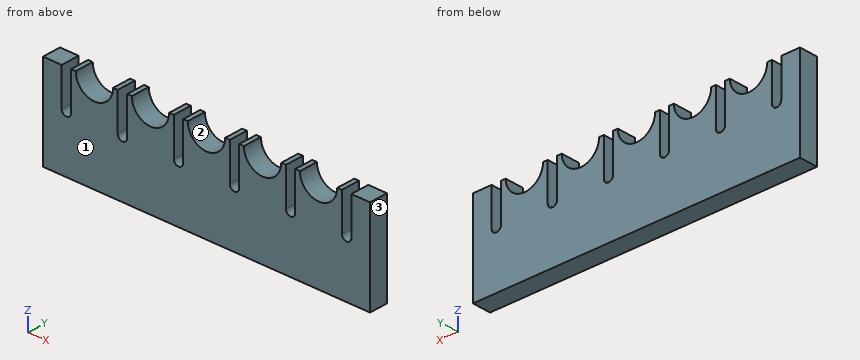
from build123d import *

# Parameters (mm, degrees)
BOSS_EXTRUDE1_DEPTH = 10


with BuildPart() as part:
    # Sketch2 → Boss-Extrude1 (new body)
    with BuildSketch(Plane(origin=(0, 0, 0), x_dir=(1, 0, 0), z_dir=(0, 1, 0))):
        with BuildLine():
            Line((-77.5, -25), (-77.5, -5))
            ThreePointArc((-77.5, -5), (-75, -2.5), (-72.5, -5))
            Line((-72.5, -5), (-72.5, -25))
            Line((-72.5, -25), (-70, -25))
            ThreePointArc((-70, -25), (-60, -15), (-50, -25))
            Line((-50, -25), (-47.5, -25))
            Line((-47.5, -25), (-47.5, -5))
            ThreePointArc((-47.5, -5), (-45, -2.5), (-42.5, -5))
            Line((-42.5, -5), (-42.5, -25))
            Line((-42.5, -25), (-40, -25))
            ThreePointArc((-40, -25), (-30, -15), (-20, -25))
            Line((-20, -25), (-17.5, -25))
            Line((-17.5, -25), (-17.5, -5))
            ThreePointArc((-17.5, -5), (-15, -2.5), (-12.5, -5))
            Line((-12.5, -5), (-12.5, -25))
            Line((-12.5, -25), (-10, -25))
            ThreePointArc((-10, -25), (0, -15), (10, -25))
            Line((10, -25), (12.5, -25))
            Line((12.5, -25), (12.5, -5))
            ThreePointArc((12.5, -5), (15, -2.5), (17.5, -5))
            Line((17.5, -5), (17.5, -25))
            Line((17.5, -25), (20, -25))
            ThreePointArc((20, -25), (30, -15), (40, -25))
            Line((40, -25), (42.5, -25))
            Line((42.5, -25), (42.5, -5))
            ThreePointArc((42.5, -5), (45, -2.5), (47.5, -5))
            Line((47.5, -5), (47.5, -25))
            Line((47.5, -25), (50, -25))
            ThreePointArc((50, -25), (60, -15), (70, -25))
            Line((70, -25), (72.5, -25))
            Line((72.5, -25), (72.5, -5))
            ThreePointArc((72.5, -5), (75, -2.5), (77.5, -5))
            Line((77.5, -5), (77.5, -25))
            Line((77.5, -25), (87.5, -25))
            Line((87.5, -25), (87.5, 25))
            Line((87.5, 25), (-87.5, 25))
            Line((-87.5, 25), (-87.5, -25))
            Line((-87.5, -25), (-77.5, -25))
        make_face()
    extrude(amount=BOSS_EXTRUDE1_DEPTH)


solid = part.part
For this review, take the finished solid that the model builds, in its own axes (mm). Face numbers are marked on the shaded views. Round coordinates to 2 decimals unless told otherwise and drop trailing zeros. Order: outer loops, then holes, each group sorted by start corner. A loop starts at its lowest first (then second) coordinate and runs counter-clockwise, first axis right, second up. Notation, with made-up numbers: (72.25, 41.5) -> (131.25, 41.5) arc R22 cw to (131.25, 51.5) -> close; hole circle Ø8 at (-37, -31). An arc over 180 degrees is marked (long way). Put each result on its own line as item: value.
Q1. Add section C-C on x = 75. Write out the cut boundary in (y, z).
Check result:
outline: (0, -25) -> (10, -25) -> (10, 2.5) -> (0, 2.5) -> close
Q2. Add section A-A on x = 30. Write out the cut boundary in (y, z), plus the area to 3 significant figures.
Check result:
outline: (0, -25) -> (10, -25) -> (10, 15) -> (0, 15) -> close
area: 400 mm2
Q3. Add section B-B on z = 20. State how many separate pieces and enclosed holes the cut face has, plus the area to 3 significant figures.
Check result:
separate pieces: 12
enclosed holes: 0
area: 584 mm2
Q4. Insertion check: pin 1 Ø2 at (x, y) = (1, 7.5) entering from +Z. The pin has a flat end and moves straight along its axis. Give the tip position at first contact, or say it passes through.
Check result:
pin 1: z = 15.2
Q5. Mouldability with a two-part tool opening along X and no side actions: class the marked faces 1, 2 and 3 as pulls with the +X half, pulls with the -X half, needs draft (parallel to the pull), parting line crosses it, or undercut.
Check result:
face 1: needs draft
face 2: undercut
face 3: pulls with the +X half
Q6. For probe 1 along Z at (x, y) = (-29.5, 2); probe 2 along Z at (x, y) = (73.5, 3), list the stretches that pass through material, from the lowest coordinate up. Write a range as [from, to].
Check result:
probe 1: [-25, 15.01]
probe 2: [-25, 3]
